Part print with two shaded views. Sizes in mm from the minimum x, y, z corner. Give positions to 0.01 mm unless a question says otherwise; leave off trailing zeros. Order: outer loops, then holes, each group sorted by start corner. A loop starts at its lowest first (then second) coordinate and runs counter-clockwise, first axis right, second up. Notation, with made-up numbers: (32.5, -5) -> (59.5, -5) arc R28 ccw to (59.5, 32) -> close; hole circle Ø5 at (28.5, 19.5). An arc over 180 degrees is marked (long way). Answer as CSV lines item,"result".
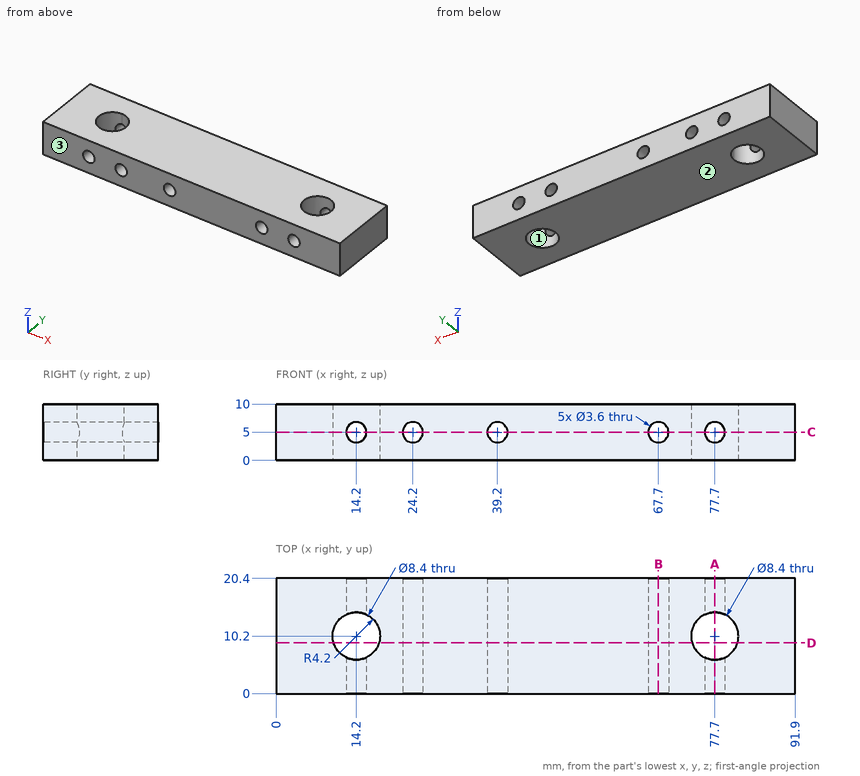
1) Band-saw the part on C-C, the plane z = 5. Give the number of separate pieces and of enclosed holes in the cut face, then the cut area to 3 significant figures.
Data:
separate pieces,"6"
enclosed holes,"0"
area,"1,460 mm2"
2) Pull direction Y, two halves, no side cores. Call the marked faces 1, 2 and 3: pulls with the +Y half, pulls with the -Y half, needs draft (parallel to the pull), parting line crosses it, or undercut.
Data:
face 1,"undercut"
face 2,"needs draft"
face 3,"pulls with the -Y half"
3) Band-saw the part on D-D, the plane y = 9. Write the cut outline in (x, z).
Data:
outline,"(0, 0) -> (10.18, 0) -> (10.18, 10) -> (0, 10) -> close; (18.22, 0) -> (73.68, 0) -> (73.68, 10) -> (18.22, 10) -> close; (81.72, 0) -> (91.9, 0) -> (91.9, 10) -> (81.72, 10) -> close; hole circle Ø3.6 at (24.2, 5); hole circle Ø3.6 at (39.2, 5); hole circle Ø3.6 at (67.7, 5)"
4) Band-saw the part on B-B, the plane x = 67.7. Write the cut outline in (y, z), then the cut area to 3 significant figures.
Data:
outline,"(0, 0) -> (20.4, 0) -> (20.4, 3.2) -> (0, 3.2) -> close; (0, 6.8) -> (20.4, 6.8) -> (20.4, 10) -> (0, 10) -> close"
area,"131 mm2"
5) Pin check, flat tip, straight feed: P1, Ø2, axis at y = 5, z = 6.5, coming from the -X side. Stop position of the tip, or through.
Data:
P1,"stops at x = 0"
6) Band-saw the part on A-A, the plane x = 77.7. Write the cut outline in (y, z).
Data:
outline,"(0, 0) -> (6, 0) -> (6, 3.2) -> (0, 3.2) -> close; (0, 6.8) -> (6, 6.8) -> (6, 10) -> (0, 10) -> close; (14.4, 0) -> (20.4, 0) -> (20.4, 3.2) -> (14.4, 3.2) -> close; (14.4, 6.8) -> (20.4, 6.8) -> (20.4, 10) -> (14.4, 10) -> close"
7) Wall check: line 1 along Z through (x, y) = (77.7, 4.25); line 2 along X through (y, z) = (7.5, 6); line 3 along Z through (x, y) = (78.5, 15). Give the ranges that are in metal, low to high. Write a range as [from, to].
Data:
line 1,"z = [0, 3.2], [6.8, 10]"
line 2,"x = [0, 10.98], [17.42, 22.7], [25.7, 37.7], [40.7, 66.2], [69.2, 74.48], [80.92, 91.9]"
line 3,"z = [0, 3.39], [6.61, 10]"
